from build123d import *

# Parameters (mm, degrees)
SKETCH013_W   = 10.8
SKETCH013_H   = 12.5
PAD072_DEPTH  = 0.3
SKETCH014_W   = 0.3
SKETCH014_H   = 12.5
PAD073_DEPTH  = 7
SKETCH015_R   = 4.15
SKETCH015_R_2 = 1.65
PAD074_DEPTH  = 8.5
CHAMFER_SIZE  = 4
FILLET_R      = 1


with BuildPart() as part:
    # Sketch013 → Pad072 (new body)
    with BuildSketch(Plane(origin=(0, -0.3, 0), x_dir=(-1, 0, 0), z_dir=(0, 1, 0))):
        Rectangle(SKETCH013_W, SKETCH013_H)
    extrude(amount=PAD072_DEPTH)

    # Sketch014 → Pad073 (join)
    with BuildSketch(Plane.XZ):
        with Locations((5.25, 0)):
            Rectangle(SKETCH014_W, SKETCH014_H)
        with Locations((-5.25, 0)):
            Rectangle(SKETCH014_W, SKETCH014_H)
    extrude(amount=-PAD073_DEPTH)

    # Sketch015 → Pad074 (join)
    with BuildSketch(Plane(origin=(0, -0.3, 0), x_dir=(-1, 0, 0), z_dir=(0, 1, 0))):
        Circle(SKETCH015_R)
        Circle(SKETCH015_R_2, mode=Mode.SUBTRACT)
    extrude(amount=-PAD074_DEPTH)

    # Chamfer
    chamfer_edges = [part.edges().sort_by_distance(p)[0] for p in [
        (-5.25, 7, 6.25),
        (5.25, 7, 6.25),
    ]]
    chamfer(chamfer_edges, length=CHAMFER_SIZE)

    # Fillet
    fillet_edges = [part.edges().sort_by_distance(p)[0] for p in [
        (4.15, -8.8, 0),
        (1.65, -8.8, 0),
    ]]
    fillet(fillet_edges, radius=FILLET_R)


with BuildPart() as part_1:
    # Pad019Body placement: moved
    add(part.part.moved(Location((28.1, 0, 6.25))))


solid = part_1.part
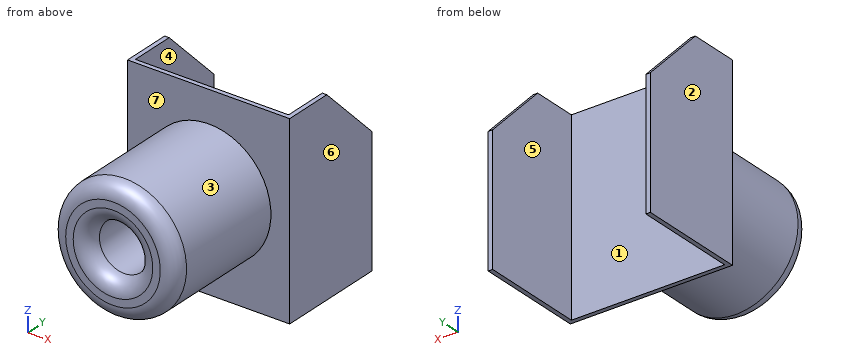
Work out the finished part from the listing and answer in its coordinate system (mm). Face numbers are marked on the shaded views. A direction names the side the tool comes from. Give positions to 0.01 mm unless a question says otherwise; leave off trailing zeros. Loops run counter-clockwise (first coordinate to the right, second up) from the corner with the lowest first, then second, coordinate; pieces in that order, holes last. Notation, with made-up numbers: (-10, 26) -> (20, 26) arc R12 ccw to (20, 41) -> close; hole circle Ø11 at (14.25, 10). An arc over 180 degrees is marked (long way). Use a Markdown table: item, result. Add a question column.
1) The part is cut by section D-D, the plane y = 6. Determine the outline of the cut face in (x, z).
2) Each of these flat-tipped pins is pushed along its axis until it touches: P1, Ø5.5, axis at x = 30, z = 9, coming from the -Y side; P2, Ø5, axis at x = 28, z = 9, coming from the +Y side; P3, Ø4, axis at y = -3, z = 2.5, coming from the +X side; P4, Ø3, axis at y = -4.5, z = 2, coming from the +X side. Where does it stop, or does it pass through?
3) The part is cut by section A-A, the plane y = 4. Determine the outline of the cut face in (x, z).
4) Consider line 1 along X through (y, z) = (5.75, 4.75); line 2 along Z through (x, y) = (28.1, -2.5); line 3 along Y through (x, z) = (32.5, 6.5). Determine where each line is inside the solid, lowest interval first.
5) For a pull along X with two mould halves and no side action, classify the marked faces 4, 5, 6 and 7 as +X half, -X half, draft (parallel to the pull), parting line (faces both ways), or undercut.
6) Which of the six approach directions +Z, -Z, +X, -X, +Y, -Y give full straight-line access (tool end or side, diameter ignored) to the marked faces 1, 2 and 3?
7) The part is cut by section B-B, the plane z = 6.25. Determine the outline of the cut face in (x, y), plus the area to 3 significant figures.
8) The part is cut by section C-C, the plane x = 28.1. Determine the outline of the cut face in (y, z).
Reported:
| question | item | result |
|---|---|---|
| 1 | outline | (22.7, 0) -> (23, 0) -> (23, 9.5) -> (22.7, 9.5) -> close; (33.2, 0) -> (33.5, 0) -> (33.5, 9.5) -> (33.2, 9.5) -> close |
| 2 | P1 | stops at y = -8.8 |
| 2 | P2 | stops at y = 0 |
| 2 | P3 | stops at x = 31.86 |
| 2 | P4 | stops at x = 31.21 |
| 3 | outline | (22.7, 0) -> (23, 0) -> (23, 11.5) -> (22.7, 11.5) -> close; (33.2, 0) -> (33.5, 0) -> (33.5, 11.5) -> (33.2, 11.5) -> close |
| 4 | line 1 | x = 22.7 to 23, 33.2 to 33.5 |
| 4 | line 2 | z = 2.1 to 4.6, 7.9 to 10.4 |
| 4 | line 3 | y = -0.3 to 0 |
| 5 | face 4 | undercut |
| 5 | face 5 | undercut |
| 5 | face 6 | +X half |
| 5 | face 7 | draft |
| 6 | face 1 | +Z, -Z, +Y |
| 6 | face 2 | +Z, -Z, -X, +Y, -Y |
| 6 | face 3 | -Y |
| 7 | outline | (22.7, -0.3) -> (23.95, -0.3) -> (23.95, -7.8) arc R1 ccw to (24.95, -8.8) -> (25.45, -8.8) arc R1 ccw to (26.45, -7.8) -> (26.45, -0.3) -> (29.75, -0.3) -> (29.75, -7.8) arc R1 ccw to (30.75, -8.8) -> (31.25, -8.8) arc R1 ccw to (32.25, -7.8) -> (32.25, -0.3) -> (33.5, -0.3) -> (33.5, 7) -> (33.2, 7) -> (33.2, 0) -> (23, 0) -> (23, 7) -> (22.7, 7) -> close |
| 7 | area | 49.1 mm^2 |
| 8 | outline | (-8.8, 3.1) arc R1 ccw to (-7.8, 2.1) -> (-0.3, 2.1) -> (-0.3, 0) -> (0, 0) -> (0, 12.5) -> (-0.3, 12.5) -> (-0.3, 10.4) -> (-7.8, 10.4) arc R1 ccw to (-8.8, 9.4) -> (-8.8, 8.9) arc R1 ccw to (-7.8, 7.9) -> (-0.3, 7.9) -> (-0.3, 4.6) -> (-7.8, 4.6) arc R1 ccw to (-8.8, 3.6) -> close |
